```python
from build123d import *

# Parameters (mm, degrees)
SKETCH1_W             = 15.1
SKETCH1_H             = 10.1
BOSS_EXTRUDE1_DEPTH   = 1.68
SKETCH3_R             = 3.34
BOSS_EXTRUDE2_DEPTH   = 1.28
FILLET1_R             = 1
M5X0_8_TAPPED_HOLE1_D = 4.2
FILLET2_R             = 1
FILLET3_R             = 0.1


with BuildPart() as part:
    # Sketch1 → Boss-Extrude1 (new body)
    with BuildSketch(Plane(origin=(0, 0, 0), x_dir=(0, 0, -1), z_dir=(1, 0, 0))):
        Rectangle(SKETCH1_W, SKETCH1_H)
    extrude(amount=BOSS_EXTRUDE1_DEPTH)

    # Sketch3 → Boss-Extrude2 (add)
    with BuildSketch(Plane(origin=(1.68, 0, 0), x_dir=(0, 0, -1), z_dir=(1, 0, 0))):
        with Locations(Location((0, 0, 0), (0, 0, 180))):
            Circle(SKETCH3_R)
    extrude(amount=BOSS_EXTRUDE2_DEPTH)

    # Fillet1
    fillet1_edges = [part.edges().sort_by_distance(p)[0] for p in [
        (2.96, 0, -3.34),
    ]]
    fillet(fillet1_edges, radius=FILLET1_R)

    # M5x0.8 Tapped Hole1 (through all)
    with Locations(Plane(origin=(2.96, 0, 0), x_dir=(0, 0, -1), z_dir=(1, 0, 0))):
        with Locations((0, 0)):
            Hole(M5X0_8_TAPPED_HOLE1_D / 2)

    # Fillet2
    fillet2_edges = [part.edges().sort_by_distance(p)[0] for p in [
        (0.84, 5.05, 7.55),
        (0.84, 5.05, -7.55),
        (0.84, -5.05, -7.55),
        (0.84, -5.05, 7.55),
    ]]
    fillet(fillet2_edges, radius=FILLET2_R)

    # Fillet3
    fillet3_edges = [part.edges().sort_by_distance(p)[0] for p in [
        (1.68, 0, -3.34),
        (0, 0, -2.1),
        (0, -5.05, 0),
        (1.68, -5.05, 0),
        (0, 0, 7.55),
        (0, 5.05, 0),
        (0, 0, -7.55),
        (0, 4.757106781, 7.257106781),
        (0, 4.757106781, -7.257106781),
        (0, -4.757106781, -7.257106781),
        (0, -4.757106781, 7.257106781),
        (1.68, 0, 7.55),
        (1.68, 0, -7.55),
        (1.68, 5.05, 0),
        (1.68, 4.757106781, 7.257106781),
        (1.68, 4.757106781, -7.257106781),
        (1.68, -4.757106781, -7.257106781),
        (1.68, -4.757106781, 7.257106781),
    ]]
    fillet(fillet3_edges, radius=FILLET3_R)


solid = part.part
```
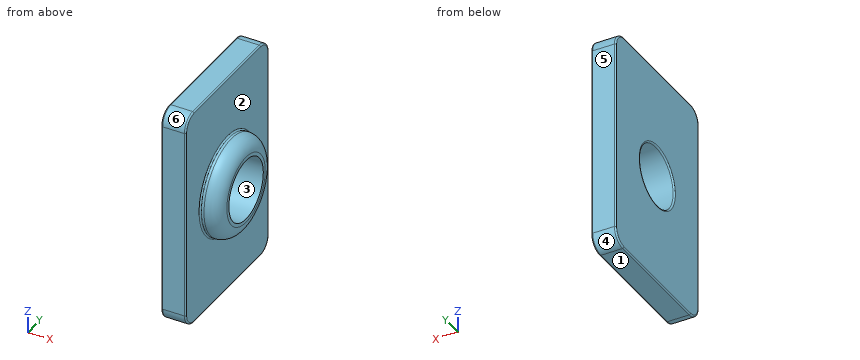
Part model, mm, in its own coordinate system. Face numbers are marked on the shaded views. A direction names the side the tool comes from. Round coordinates to 2 decimals unless told otherwise and drop trailing zeros. Loops run counter-clockwise (first coordinate to the right, second up) from the corner with the lowest first, then second, coordinate; pieces in that order, holes last.
1. 3-axis set-ups, long thin cutter, end or side, ignore diameter. For the marked faces 1 and 2: which of +Z, -Z, +X, -X, +Y, -Y reach the whole face in a straight line?
Solutions:
face 1: -Z, +X, -X, +Y, -Y
face 2: +X
2. Slice it at B-B (y = 0). Give the cut face in (x, z), and give its area (3 significant figures).
Solutions:
outline: (0, -7.45) arc R0.1 ccw to (0.1, -7.55) - (1.58, -7.55) arc R0.1 ccw to (1.68, -7.45) - (1.68, -3.44) arc R0.1 cw to (1.78, -3.34) - (1.96, -3.34) arc R1 ccw to (2.96, -2.34) - (2.96, -2.1) - (0.1, -2.1) arc R0.1 ccw to (0, -2.2) - close; (0, 2.2) arc R0.1 ccw to (0.1, 2.1) - (2.96, 2.1) - (2.96, 2.34) arc R1 ccw to (1.96, 3.34) - (1.78, 3.34) arc R0.1 cw to (1.68, 3.44) - (1.68, 7.45) arc R0.1 ccw to (1.58, 7.55) - (0.1, 7.55) arc R0.1 ccw to (0, 7.45) - close
area: 21.0 mm2
3. Slice it at D-D (z = 4.5). Give the cut face in (x, y), and give its area (3 significant figures).
Solutions:
outline: (0, -4.95) arc R0.1 ccw to (0.1, -5.05) - (1.58, -5.05) arc R0.1 ccw to (1.68, -4.95) - (1.68, 4.95) arc R0.1 ccw to (1.58, 5.05) - (0.1, 5.05) arc R0.1 ccw to (0, 4.95) - close
area: 17.0 mm2
4. Drill centre lines: line 1 along Y through (x, z) = (0.7, 0); line 2 along X through (y, z) = (-2, -6.5); line 3 along Z through (x, y) = (0.6, 1). Where is each one in solid material? Low to high.
Solutions:
line 1: y = -5.05 to -2.1, 2.1 to 5.05
line 2: x = 0 to 1.68
line 3: z = -7.55 to -1.85, 1.85 to 7.55
5. Flat gauge pin, fed straight in: pin 1 (1.5 mm diameter, centred on y = -3.5, z = -1.5, fed in from +X). Where does the tip first touch, or does it go through?
Solutions:
pin 1: stops at x = 2.66
6. Two-plate mould, pull along Z, no slides. Class the marked faces 3, 4, 5 and 6: pulls with the +Z half, pulls with the -Z half, needs draft (parallel to the pull), parting line crosses it, or undercut.
Solutions:
face 3: undercut
face 4: pulls with the -Z half
face 5: needs draft
face 6: pulls with the +Z half
7. Slice it at A-A (z = 0). Give the cut face in (x, y).
Solutions:
outline: (0, -4.95) arc R0.1 ccw to (0.1, -5.05) - (1.58, -5.05) arc R0.1 ccw to (1.68, -4.95) - (1.68, -3.44) arc R0.1 cw to (1.78, -3.34) - (1.96, -3.34) arc R1 ccw to (2.96, -2.34) - (2.96, -2.1) - (0.1, -2.1) arc R0.1 ccw to (0, -2.2) - close; (0, 2.2) arc R0.1 ccw to (0.1, 2.1) - (2.96, 2.1) - (2.96, 2.34) arc R1 ccw to (1.96, 3.34) - (1.78, 3.34) arc R0.1 cw to (1.68, 3.44) - (1.68, 4.95) arc R0.1 ccw to (1.58, 5.05) - (0.1, 5.05) arc R0.1 ccw to (0, 4.95) - close
8. Slice it at C-C (x = 0.35). Give the cut face in (y, z), and give its area (3 significant figures).
Solutions:
outline: (-5.05, -6.55) arc R1 ccw to (-4.05, -7.55) - (4.05, -7.55) arc R1 ccw to (5.05, -6.55) - (5.05, 6.55) arc R1 ccw to (4.05, 7.55) - (-4.05, 7.55) arc R1 ccw to (-5.05, 6.55) - close; hole circle Ø4.2 at (0, 0)
area: 138 mm2
